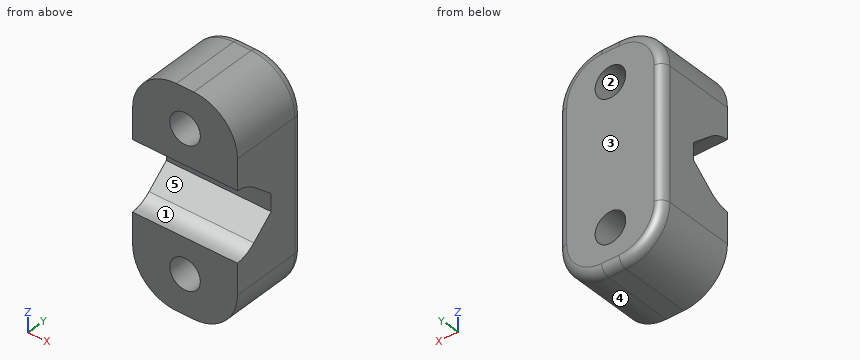
```python
from build123d import *

# Parameters (mm, degrees)
CROQUIS1_W              = 12
CROQUIS1_H              = 25
SALIENTE_EXTRUIR1_DEPTH = 9
CORTAR_EXTRUIR1_DEPTH   = 13
CROQUIS4_R              = 1.75
CORTAR_EXTRUIR2_DEPTH   = 10
REDONDEO1_R             = 5
REDONDEO2_R             = 1


with BuildPart() as part:
    # Croquis1 → Saliente-Extruir1 (new body)
    with BuildSketch(Plane(origin=(0, 0, 0), x_dir=(1, 0, 0), z_dir=(0, 1, 0))):
        with Locations((6, 0)):
            Rectangle(CROQUIS1_W, CROQUIS1_H)
    extrude(amount=SALIENTE_EXTRUIR1_DEPTH)

    # Croquis3 → Cortar-Extruir1 (cut, through all)
    with BuildSketch(Plane(origin=(0, 0, 0), x_dir=(0, 0, -1), z_dir=(1, 0, 0))):
        with BuildLine():
            Line((-3.047905892, 2.290418822), (-1, 4.7))
            Line((-1, 4.7), (1, 4.7))
            Line((1, 4.7), (3.047905892, 2.290418822))
            ThreePointArc((3.047905892, 2.290418822), (0, -4.3), (-3.047905892, 2.290418822))
        make_face()
    extrude(amount=CORTAR_EXTRUIR1_DEPTH, mode=Mode.SUBTRACT)

    # Croquis4 → Cortar-Extruir2 (cut, through all)
    with BuildSketch(Plane.XZ):
        with Locations((6, 8)):
            Circle(CROQUIS4_R)
        with Locations((6, -8)):
            Circle(CROQUIS4_R)
    extrude(amount=-CORTAR_EXTRUIR2_DEPTH, mode=Mode.SUBTRACT)

    # Redondeo1
    redondeo1_edges = [part.edges().sort_by_distance(p)[0] for p in [
        (0, 4.5, -12.5),
        (12, 4.5, -12.5),
        (12, 4.5, 12.5),
        (0, 4.5, 12.5),
    ]]
    fillet(redondeo1_edges, radius=REDONDEO1_R)

    # Redondeo2
    redondeo2_edges = [part.edges().sort_by_distance(p)[0] for p in [
        (0, 9, 0),
        (6, 9, -12.5),
        (6, 9, 12.5),
        (12, 9, 0),
        (1.464466094, 9, 11.035533906),
        (10.535533906, 9, 11.035533906),
        (10.535533906, 9, -11.035533906),
        (1.464466094, 9, -11.035533906),
    ]]
    fillet(redondeo2_edges, radius=REDONDEO2_R)


solid = part.part
```
The model under review builds one solid part; all positions refer to its coordinate system, in mm. Face numbers are marked on the shaded views. A direction names the side the tool comes from. Round coordinates to 2 decimals unless told otherwise and drop trailing zeros. Loops run counter-clockwise (first coordinate to the right, second up) from the corner with the lowest first, then second, coordinate; pieces in that order, holes last. Notation, with made-up numbers: M 67,57.25 L 80,57.25 A36 ccw 80,91.25 Z; hole C 14.5,-36 d10. An arc over 180 degrees is marked long. Write item = value, one per line.
Item 1: The part is to be moulded in two halves that separate along Z. For the marked faces 3, 4 and 5, say which applies: released by +Z, released by -Z, zero draft, split by the parting line, or undercut.
Return value:
face_3 = zero draft
face_4 = released by -Z
face_5 = undercut
Item 2: Take a section at A-A on x = 6. Write out the cut boundary in (y, z), then the cut area to 3 significant figures.
Return value:
outline = M 0,-12.5 L 8,-12.5 A1 ccw 9,-11.5 L 9,-9.75 L 0,-9.75 Z; M 0,-6.25 L 9,-6.25 L 9,6.25 L 0,6.25 L 0,3.99 A4 cw 2.29,3.05 L 4.7,1 L 4.7,-1 L 2.29,-3.05 A4 cw 0,-3.99 Z; M 0,9.75 L 9,9.75 L 9,11.5 A1 ccw 8,12.5 L 0,12.5 Z
area = 135 mm2
Item 3: Take a section at D-D on z = -0.5. Write out the cut boundary in (x, y).
Return value:
outline = M 0,4.7 L 12,4.7 L 12,8 A1 ccw 11,9 L 1,9 A1 ccw 0,8 Z
Item 4: For line 1 (Z direction, x = 6, y = 5.5); line 2 (Z direction, x = 6, y = 0.75); line 3 (Z direction, x = 5, y = 2.5), list the stretches that pass through material, from the lowest coordinate up. Write a range as [from, to].
Return value:
line_1 = [-12.5, -9.75], [-6.25, 6.25], [9.75, 12.5]
line_2 = [-12.5, -9.75], [-6.25, -3.86], [3.86, 6.25], [9.75, 12.5]
line_3 = [-12.5, -9.44], [-6.56, -2.87], [2.87, 6.56], [9.44, 12.5]
Item 5: Take a section at B-B on y = 2.75. Write out the cut boundary in (x, z).
Return value:
outline = M 0,-7.5 A5 ccw 5,-12.5 L 7,-12.5 A5 ccw 12,-7.5 L 12,-2.66 L 0,-2.66 Z; M 0,2.66 L 12,2.66 L 12,7.5 A5 ccw 7,12.5 L 5,12.5 A5 ccw 0,7.5 Z; hole C 6,-8 d3.5; hole C 6,8 d3.5
Item 6: Take a section at C-C on y = 6.5. Write out the cut boundary in (x, z), then the cut area to 3 significant figures.
Return value:
outline = M 0,-7.5 A5 ccw 5,-12.5 L 7,-12.5 A5 ccw 12,-7.5 L 12,7.5 A5 ccw 7,12.5 L 5,12.5 A5 ccw 0,7.5 Z; hole C 6,-8 d3.5; hole C 6,8 d3.5
area = 259 mm2
Item 7: Insertion check: P1, Ø2, axis at x = 2.5, z = 1.5, coming from the -Y side; P2, Ø1.6, axis at x = 5.5, z = 0, coming from the -Y side. Each pin has a flat end and moves straight along its axis. Give the tip position at first contact, or say it passes through.
Return value:
P1 = 2.94
P2 = 4.7
Item 8: Machinability: for the marked faces 1 and 2, which of the approach directions +Z, -Z, +X, -X, +Y, -Y give a long, thin tool a straight path to every point of the face, cutting with its end or side? Answer none if there is none.
Return value:
face_1 = +X, -X, -Y
face_2 = +Y, -Y
